Check sheet for the modelled part. Datum: model origin and axes. Units: mm. Round coordinates to 2 decimals unless told otherwise and drop trailing zeros. Write each loop counter-clockwise with the first axis right and the second up, starting at its lowest first coordinate (ties: lowest second). Pieces come first, ordered by that corner, then holes.
Item 1: Cross-section at C-C on x = 0. Enter the section's corners in (y, z).
Item 2: Cross-section at A-A on y = 0. Enter the section's corners in (x, z), plus the area to 3 significant figures.
Item 3: Cross-section at B-B on x = 6.5. Enter the section's corners in (y, z), plus the area to 3 significant figures.
Item 4: Release check for a two-part mould opening along X. For faces 1 (the cylindrical face through (-8.771, -8.043, 2.465)), 2 (the flat face through (12.4, 0.3, 0)), 3 (the cylindrical face through (-12.574, -8.99, 2.465)), 4 (the cylindrical face through (8.767, 16.856, 2.465)) record: +X half, -X half, draft (parallel to the pull), parting line (faces both ways), or undercut.
Item 5: Material ranges on line 1 (Y direction, x = 0, z = 3.1); line 2 (X direction, y = -7, z = 3.3); line 3 (X direction, y = 7, z = 2.8), recorded low to high.
Item 6: Cross-section at D-D on y = -7. Enter the section's corners in (x, z).
Item 7: Go/stop test with flat-tipped pins: pin 1 Ø3 at (x, z) = (9, 1.5) entering from +Y; pin 2 Ø1.5 at (x, z) = (-2, 0.5) entering from +Y; pin 3 Ø3.5 at (x, y) = (13.38, -7.72) entering from +Z; pin 4 Ø1 at (x, z) = (11.5, 4) entering from +Y. Record where each tip stops, or that it passes through.
Autodesk Inventor part; units mm, degrees
ref_plane "YZ Plane" through (0, 0, 0) normal (1, 0, 0) x (0, 1, 0)
ref_plane "XZ Plane" through (0, 0, 0) normal (0, 1, 0) x (-1, 0, 0)
ref_plane "XY Plane" through (0, 0, 0) normal (0, 0, 1) x (1, 0, 0)
ref_plane "РабПлоскость1" through (0, 0, 0) normal (0, 0, 1) x (1, 0, 0)
sketch "Эскиз1" plane through (0, 0, 0) normal (0, 0, 1) x (1, 0, 0)
  circle A0 centre (0, 0) radius 11.9
  circle A1 centre (0, 0) radius 19
  circle A2 centre (-13.3801, -7.725) radius 1.5
  circle A3 centre (13.3801, -7.725) radius 1.5
  circle A4 centre (0, 15.45) radius 1.5
  dimension "d12" = 3
  dimension "d13" = 3
  dimension "d14" = 3
extrude "Выдавливание1" add sketch "Эскиз1" along normal blind 5
properties part number "Проставка шестерни"
Response values:
1. outline: (-19, 0) - (-11.9, 0) - (-11.9, 5) - (-19, 5) - close; (11.9, 0) - (13.95, 0) - (13.95, 5) - (11.9, 5) - close; (16.95, 0) - (19, 0) - (19, 5) - (16.95, 5) - close
2. outline: (-19, 0) - (-11.9, 0) - (-11.9, 5) - (-19, 5) - close; (11.9, 0) - (19, 0) - (19, 5) - (11.9, 5) - close
2. area: 71.0 mm2
3. outline: (-17.85, 0) - (-9.97, 0) - (-9.97, 5) - (-17.85, 5) - close; (9.97, 0) - (17.85, 0) - (17.85, 5) - (9.97, 5) - close
3. area: 78.9 mm2
4. face 1: undercut
4. face 2: draft
4. face 3: undercut
4. face 4: parting line
5. line 1: y = -19 to -11.9, 11.9 to 13.95, 16.95 to 19
5. line 2: x = -17.66 to -14.69, -12.07 to -9.62, 9.62 to 12.07, 14.69 to 17.66
5. line 3: x = -17.66 to -9.62, 9.62 to 17.66
6. outline: (-17.66, 0) - (-14.69, 0) - (-14.69, 5) - (-17.66, 5) - close; (-12.07, 0) - (-9.62, 0) - (-9.62, 5) - (-12.07, 5) - close; (9.62, 0) - (12.07, 0) - (12.07, 5) - (9.62, 5) - close; (14.69, 0) - (17.66, 0) - (17.66, 5) - (14.69, 5) - close
7. pin 1: stops at y = 17.46
7. pin 2: stops at y = 18.96
7. pin 3: stops at z = 5
7. pin 4: stops at y = 15.49
